Build history of the part. All positions in model axes, mm. Face numbers are marked on the shaded views. A direction names the side the tool comes from. Round coordinates to 2 decimals unless told otherwise and drop trailing zeros. Write each loop counter-clockwise with the first axis right and the second up, starting at its lowest first coordinate (ties: lowest second). Pieces come first, ordered by that corner, then holes. Notation, with made-up numbers: (79.5, 26.25) -> (115.5, 26.25) arc R8 cw to (115.5, 32.25) -> close; hole circle Ø6 at (-7.5, 68). An arc over 180 degrees is marked (long way). Answer in a Markdown table with one row per item.
```python
from build123d import *


with BuildPart() as f1:
    # F0 (on Top) → F1 (revolve)
    with BuildSketch(Plane.XY):
        with BuildLine():
            ThreePointArc((-18.994163, 13.121947), (-18.526276, 29.537549), (-32.016402, 20.172325))
            ThreePointArc((-32.016402, 20.172325), (-34.616866, 15.535363), (-36.593492, 10.600104))
            Line((-36.593492, 10.600104), (-28.713267, 0))
            Line((-28.713267, 0), (-36.593492, -14.794178))
            Line((-36.593492, -14.794178), (-23.228711, -14.794178))
            Line((-23.228711, -14.794178), (-18.296746, -6.879023))
            Line((-18.296746, -6.879023), (-5.593964, -14.794178))
            Line((-5.593964, -14.794178), (0, -14.794178))
            Line((0, -14.794178), (0, -7.429056))
            Line((0, -7.429056), (-22.906089, 6.84382))
            Line((-22.906089, 6.84382), (-18.994163, 13.121947))
        make_face()
    revolve(axis=Axis((0, -11.111617, 0), (0, -1, 0)))


solid = f1.part
```
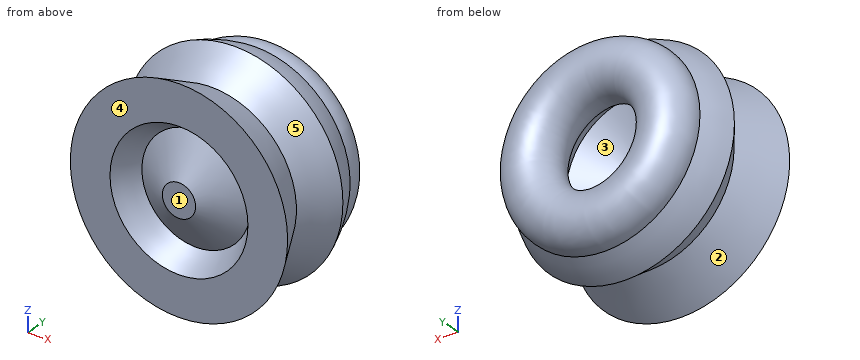
Q1. Two-plate mould, pull along Z, no slides. Class the marked faces 1, 2 and 3: released by +Z, released by -Z, zero draft, split by the parting line, or undercut.
A:
| item | result |
|---|---|
| face 1 | zero draft |
| face 2 | split by the parting line |
| face 3 | undercut |
Q2. Which spindle directions (+Z, -Z, +X, -X, +Y, -Y) get a long thin tool onto all of the face, cutting with end or side? Do the marked faces 4 and 5. Say none if no direction does.
A:
| item | result |
|---|---|
| face 4 | +Z, -Z, +X, -X, -Y |
| face 5 | none |
Q3. Drop flat-ended pins along their axis: P1, Ø5, axis at x = 17, z = -3, coming from the -Y side; P2, Ø5, axis at x = 25, y = 19, coming from the -Z side; P3, Ø2, axis at x = -10.5, z = 14, coming from the -Y side. Give the stop position or say it passes through.
A:
| item | result |
|---|---|
| P1 | y = -9.23 |
| P2 | z = -24.51 |
| P3 | y = -8 |
Q4. Wall check: line 1 (Z direction, x = -3, y = -7.5); line 2 (Y direction, x = -30, z = 4.5); line 3 (Y direction, x = -27, z = -10). Give the ranges that are in metal, low to high. Write a range as [from, to].
A:
| item | result |
|---|---|
| line 1 | [-32.57, -18.44], [-17.04, 17.04], [18.44, 32.57] |
| line 2 | [-14.79, -3.05], [2.18, 26.87] |
| line 3 | [-14.79, -0.15], [0.11, 28.52] |
Q5. Saw through at B-B on y = 25.5. Write the cut outline in (x, z).
A:
| item | result |
|---|---|
| outline | circle Ø62.33 at (0, 0); hole circle Ø29.29 at (0, 0) |
Q6. Saw through at A-A on y = 9. Write the cut outline in (x, z), plus the area to 3 significant figures.
A:
| item | result |
|---|---|
| outline | circle Ø70.81 at (0, 0); hole circle Ø43.13 at (0, 0) |
| area | 2,480 mm² |
